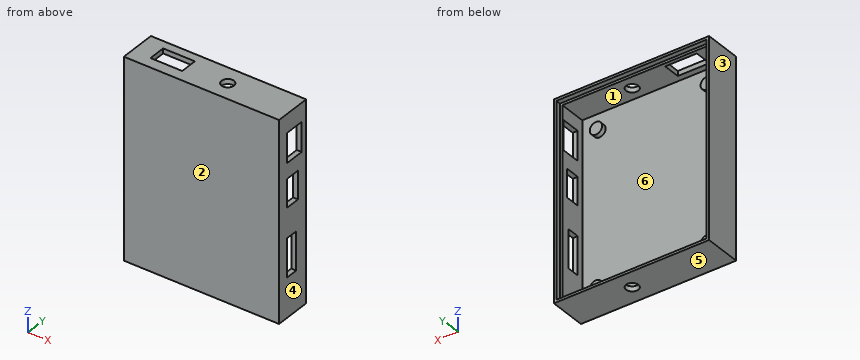
Autodesk Inventor part; units mm, degrees
ref_plane "YZ Plane" through (0, 0, 0) normal (1, 0, 0) x (0, 1, 0)
ref_plane "XZ Plane" through (0, 0, 0) normal (0, 1, 0) x (-1, 0, 0)
ref_plane "XY Plane" through (0, 0, 0) normal (0, 0, 1) x (1, 0, 0)
sketch "Sketch1" plane through (0, 0, 0) normal (0, 1, 0) x (-1, 0, 0)
  line L0 (0, 0) -> (62.86, 0)
  line L1 (62.86, 0) -> (62.86, -80.39)
  line L2 (62.86, -80.39) -> (0, -80.39)
  line L3 (0, -80.39) -> (0, 0)
  line L4 (2, -2) -> (60.86, -2)
  line L5 (60.86, -2) -> (60.86, -78.39)
  line L6 (60.86, -78.39) -> (2, -78.39)
  line L7 (2, -78.39) -> (2, -2)
  dimension "d0" = 62.86
  dimension "d1" = 80.39
  dimension "d2" = 58.86
  dimension "d3" = 76.39
  dimension "d4" = 2
  dimension "d5" = 2
extrude "Extrusion1" add sketch "Sketch1" along normal blind 15 contours L0 L1 L2 L3 | L4 L5 L6 L7
shell "Shell1" thickness 2 removed faces 1 at (-20.9533, 15, -26.7967)
sketch "Sketch2" plane through (-60.86, 2, -2) normal (0, 1, 0) x (1, 0, 0)
  point P0 (60.86, -2)
sketch "Sketch3" plane through (0, 15, 0) normal (0, 1, 0) x (1, 0, 0)
  line L0 (-60.86, 2) -> (-60.86, 78.39)
  line L1 (-60.86, 78.39) -> (-2, 78.39)
  line L2 (-2, 78.39) -> (-2, 2)
  line L3 (-2, 2) -> (-60.86, 2)
  line L4 (-62.86, 0) -> (0, 0)
  line L5 (0, 0) -> (0, 80.39)
  line L6 (0, 80.39) -> (-62.86, 80.39)
  line L7 (-62.86, 80.39) -> (-62.86, 0)
  line L8 (-61.86, 79.39) -> (-1, 79.39)
  line L9 (-1, 79.39) -> (-1, 1)
  line L10 (-1, 1) -> (-61.86, 1)
  line L11 (-61.86, 1) -> (-61.86, 79.39)
  dimension "d9" = 1
  dimension "d10" = 1
  dimension "d11" = 1
  dimension "d12" = 1
extrude "Extrusion2" cut sketch "Sketch3" against normal blind 2 contours L8 L9 L10 L11
sketch "Sketch4" plane through (-60.86, 2, -2) normal (0, 1, 0) x (1, 0, 0)
  circle A0 centre (7, 69.39) radius 2.5
  circle A1 centre (51.86, 69.39) radius 2.5
  circle A2 centre (7, 7) radius 2.5
  circle A3 centre (51.86, 7) radius 2.5
  line L0 (60.86, 78.39) -> (-2, 78.39)
  line L1 (-2, 78.39) -> (-2, -2)
  line L2 (60.86, -2) -> (60.86, 78.39)
  line L3 (-2, -2) -> (60.86, -2)
  dimension "d15" = 9
  dimension "d16" = 9
  dimension "d17" = 9
  dimension "d18" = 9
  dimension "d19" = 9
  dimension "d20" = 9
  dimension "d21" = 9
  dimension "d22" = 9
  dimension "d23" = 5
  dimension "d24" = 5
  dimension "d25" = 5
  dimension "d26" = 5
extrude "Extrusion3" add sketch "Sketch4" along normal blind 2 contours A0 | A1 | A2 | A3
sketch "Sketch5" plane through (0, 0, 0) normal (1, 0, 0) x (0, 0, -1)
  line L0 (11.5, 4) -> (6.5, 4)
  line L1 (73.89, 4) -> (68.89, 4)
  line L2 (68.89, 2) -> (68.89, 4)
  line L3 (73.89, 2) -> (73.89, 4)
  line L4 (78.39, 2) -> (2, 2)
  line L5 (78.39, 2) -> (78.39, 13)
  line L6 (80.39, 0) -> (0, 0)
  line L7 (80.39, 0) -> (80.39, 15)
  line L8 (0, 15) -> (80.39, 15)
  line L9 (0, 0) -> (0, 15)
  line L10 (11.5, 2) -> (11.5, 4)
  line L11 (2, 2) -> (2, 13)
  line L12 (6.5, 2) -> (6.5, 4)
  line L13 (79.39, 13) -> (1, 13)
  line L14 (7.5, 12.508) -> (19.3903, 12.508)
  line L15 (19.3903, 12.508) -> (19.3903, 4.508)
  line L16 (19.3903, 4.508) -> (7.5, 4.508)
  line L17 (7.5, 4.508) -> (7.5, 12.508)
  line L18 (25.6078, 10.508) -> (36.9891, 10.508)
  line L19 (36.9891, 10.508) -> (36.9891, 4.508)
  line L20 (36.9891, 4.508) -> (25.6078, 4.508)
  line L21 (25.6078, 4.508) -> (25.6078, 10.508)
  line L22 (49.0027, 9.508) -> (64.4938, 9.508)
  line L23 (64.4938, 9.508) -> (64.4938, 4.508)
  line L24 (64.4938, 4.508) -> (49.0027, 4.508)
  line L25 (49.0027, 4.508) -> (49.0027, 9.508)
  dimension "d29" = 0.508
  dimension "d30" = 8
  dimension "d31" = 6
  dimension "d32" = 5
extrude "Extrusion4" cut sketch "Sketch5" against normal blind 2 contours L14 L15 L16 L17 | L18 L19 L20 L21 | L22 L23 L24 L25
sketch "Sketch6" plane through (-62.86, 0, 0) normal (0, 0, 1) x (1, 0, 0)
  line L0 (60.86, 2) -> (2, 2)
  line L1 (11.5, 4) -> (6.5, 4)
  line L2 (11.5, 2) -> (11.5, 4)
  line L3 (6.5, 2) -> (6.5, 4)
  line L4 (60.86, 2) -> (60.86, 13)
  line L5 (56.36, 4) -> (51.36, 4)
  line L6 (51.36, 2) -> (51.36, 4)
  line L7 (56.36, 2) -> (56.36, 4)
  line L8 (2, 2) -> (2, 13)
  line L9 (61.86, 13) -> (1, 13)
  line L10 (7.5, 11.508) -> (20.3381, 11.508)
  line L11 (20.3381, 11.508) -> (20.3381, 4.508)
  line L12 (20.3381, 4.508) -> (7.5, 4.508)
  line L13 (7.5, 4.508) -> (7.5, 11.508)
  circle A0 centre (36.6004, 7.508) radius 2.5
  point P0 (62.86, 0)
  dimension "d35" = 0.508
  dimension "d36" = 7
  dimension "d37" = 5
  dimension "d38" = 5.508
extrude "Extrusion5" cut sketch "Sketch6" against normal blind 2 contours L10 L11 L12 L13 | A0
sketch "Sketch7" plane through (0, 0, -80.39) normal (0, 0, -1) x (-1, 0, 0)
  circle A0 centre (26.2596, 7.508) radius 2.5
  point P0 (0, 0)
extrude "Extrusion6" cut sketch "Sketch7" against normal blind 2
properties part number "pcbProtectiveCase"
Geometry check sheet. Reference: the model listing, model coordinates, mm. Face numbers are marked on the shaded views. A direction names the side the tool comes from. Coordinates: 2 decimals unless noted, no trailing zeros. Write each loop counter-clockwise with the first axis right and the second up, starting at its lowest first coordinate (ties: lowest second). Pieces come first, ordered by that corner, then holes. Notation, with made-up numbers: M 66.5,64 L 109.5,64 A10 cw 109.5,83 Z; hole C 81,32.25 d5. An arc over 180 degrees is marked long. Use one line per item in the form item = value. Start each with the question number.
1) Set-up check for the marked faces 5 and 6: record each of +Z, -Z, +X, -X, +Y, -Y from which the full face is reachable in a straight line by a thin tool's end or side.
2) Section check C-C on x = -20.5. Enter the section's corners in (y, z), and give its area (3 significant figures).
3) Section check A-A on z = -32. Enter the section's corners in (x, y).
4) Release check for a two-part mould opening along X. For the marked faces 1, 2, 3 and 4 record: pulls with the +X half, pulls with the -X half, needs draft (parallel to the pull), parting line crosses it, or undercut.
5) Go/stop test with flat-tipped pins: pin 1 Ø12 at (x, z) = (-35, -8.5) entering from +Y; pin 2 Ø1.5 at (x, z) = (-53.5, -71.5) entering from +Y. Record where each tip stops, or that it passes through.
6) Section check D-D on z = -9. Enter the section's corners in (x, y).
7) Section check B-B on x = -53.86. Enter the section's corners in (y, z), and give its area (3 significant figures).
8) Thickness scan on probe 1 along X at (y, z) = (13.25, -77); probe 2 along X at (y, z) = (2.25, -31); probe 3 along Z at (x, y) = (-8.5, 13.75). Record the ranges inside material, lowest first. Write a range as from..to.
Responses:
q1.face_5 = -Z, +X, -X, +Y, -Y
q1.face_6 = +Y
q2.outline = M 0,-80.39 L 15,-80.39 L 15,-79.39 L 13,-79.39 L 13,-78.39 L 2,-78.39 L 2,-2 L 13,-2 L 13,-1 L 15,-1 L 15,0 L 0,0 Z
q2.area = 209 mm2
q3.outline = M -62.86,0 L 0,0 L 0,4.51 L -2,4.51 L -2,2 L -60.86,2 L -60.86,13 L -61.86,13 L -61.86,15 L -62.86,15 Z; M -2,10.51 L 0,10.51 L 0,15 L -1,15 L -1,13 L -2,13 Z
q4.face_1 = undercut
q4.face_2 = needs draft
q4.face_3 = pulls with the -X half
q4.face_4 = pulls with the +X half
q5.pin_1 = 2
q5.pin_2 = 4
q6.outline = M -62.86,0 L 0,0 L 0,4.51 L -2,4.51 L -2,2 L -6.5,2 L -6.5,4 L -11.5,4 L -11.5,2 L -51.36,2 L -51.36,4 L -56.36,4 L -56.36,2 L -60.86,2 L -60.86,13 L -61.86,13 L -61.86,15 L -62.86,15 Z; M -2,12.51 L 0,12.51 L 0,15 L -1,15 L -1,13 L -2,13 Z
q7.outline = M 0,-80.39 L 15,-80.39 L 15,-79.39 L 13,-79.39 L 13,-78.39 L 2,-78.39 L 2,-73.89 L 4,-73.89 L 4,-68.89 L 2,-68.89 L 2,-11.5 L 4,-11.5 L 4,-6.5 L 2,-6.5 L 2,-2 L 4.51,-2 L 4.51,0 L 0,0 Z; M 11.51,-2 L 13,-2 L 13,-1 L 15,-1 L 15,0 L 11.51,0 Z
q7.area = 215 mm2
q8.probe_1 = -62.86..-61.86, -1..0
q8.probe_2 = -62.86..-60.86, -2..0
q8.probe_3 = -80.39..-79.39, -1..0
